Here's how the part is built. I have some questions about the finished solid (model axes, mm). A direction names the side the tool comes from. Give positions to 0.01 mm unless a question says otherwise; leave off trailing zeros. Loops run counter-clockwise (first coordinate to the right, second up) from the corner with the lowest first, then second, coordinate; pieces in that order, holes last. Notation, with made-up numbers: (-2.75, 36) - (45.25, 36) arc R13 cw to (45.25, 47) - close; hole circle Ø8 at (20.25, 25). An arc over 180 degrees is marked (long way). Return JSON: item names as keys, results as strings. Group by question number.
(1) For P1, Ø6, axis at x = 4.5, y = -23.5, coming from the +Z side; P2, Ø5, axis at x = -10.5, y = -39.5, coming from the +Z side; P3, Ø2.5, axis at y = -87.5, z = 10, coming from the -X side, each with a flat end and sliding along its axis, tell me the tip position at first contact or that it passes through.
(2) If we section it at D-D (y = 4.5): Please give me the cut outline in (x, z), then the cut area to 3 significant figures.
(3) If we section it at C-C (y = -60.5): Please give me the cut outline in (x, z).
(4) If we mould it in two halves opening along X, with no side actions, what happens to faces 1 (the cylindrical face through (-2.859, -21.203, 10.528)), 2 (the flat face through (-12.3, -10, -3.4)), 3 (the cylindrical face through (9.76, 34.65, -2.17)), 4 (the cylindrical face through (2.859, -21.203, 10.528))? For each: released by +X, released by -X, zero draft, split by the parting line, or undercut.
(5) I need wall thicknesses on probe 1 along Y at (x, z) = (8.75, 6); probe 2 along X at (y, z) = (-17, -0.75); probe 3 along Y at (x, z) = (-12, -8.75). Which ranges of each line are inside material? Lowest first, please. Write a range as [from, to].
(6) On a 3-axis mill with a long thin cutter (end or side, diameter ignored), from which of +Z, -Z, +X, -X, +Y, -Y can I reach the whole of each face in a straight line? I mean faces 5 (the cylindrical face through (-0.66, -0.14, -14.985)), 6 (the flat face through (4, -68, 10)), 7 (the cylindrical face through (7.606, -60.7, -9.92)), 8 (the flat face through (10, 10, -3)). Say none if no direction works.
(7) If we section it at A-A (z = 0): Please give me the cut outline in (x, y).
(8) If we section it at B-B (x = 5.75): Please give me the cut outline in (y, z).
```python
from build123d import *

# Parameters (mm, degrees)
F2_W     = 8
F2_H     = 4
F3_DEPTH = 90
F4_R     = 3.99999


# Not quite as in the source:
# - a fillet or chamfer is up to 0.001 mm smaller than in the source, because OpenCascade refuses the exact size


with BuildPart() as f1:
    # F0 (on Right) → F1 (revolve)
    with BuildSketch(Plane.YZ):
        Polygon((-110, 12.5), (-110, 0), (60, 0), (60, 10), (10, 10), (10, 15), (-10, 15), (-10, 12.5), align=None)
    revolve(axis=Axis((0, -25, 0), (0, -1, 0)))

    # F2 (on face) → F3 (cut)
    with BuildSketch(Plane.XZ.offset(110)):
        with Locations((0, 10.5)):
            Rectangle(F2_W, F2_H)
    extrude(amount=-F3_DEPTH, mode=Mode.SUBTRACT)

    # F4 (radius 4 in the source; OpenCascade refuses exactly that, so slightly less here)
    f4_edges = [f1.edges().sort_by_distance(p)[0] for p in [
        (-4, -20, 10.17136),
        (4, -20, 10.17136),
    ]]
    fillet(f4_edges, radius=F4_R)


solid = f1.part
```
Values:
{
 "1": {"P1": "z = 12.2", "P2": "z = 9.6", "P3": "x = -8.93"},
 "2": {"outline": "circle Ø30 at (0, 0)", "area": "707 mm2"},
 "3": {"outline": "(-4, 8.5) - (-4, 11.84) arc R12.5 ccw (long way) to (4, 11.84) - (4, 8.5) - close"},
 "4": {"face 1": "undercut", "face 2": "zero draft", "face 3": "split by the parting line", "face 4": "undercut"},
 "5": {"probe 1": "[-110, 10]", "probe 2": "[-12.48, 12.48]", "probe 3": "[-10, 10]"},
 "6": {"face 5": "+Y, -Y", "face 6": "+Z, -Y", "face 7": "-Y", "face 8": "+Y"},
 "7": {"outline": "(-15, -10) - (-12.5, -10) - (-12.5, -110) - (12.5, -110) - (12.5, -10) - (15, -10) - (15, 10) - (10, 10) - (10, 60) - (-10, 60) - (-10, 10) - (-15, 10) - close"},
 "8": {"outline": "(-110, -11.1) - (-10, -11.1) - (-10, -13.85) - (10, -13.85) - (10, -8.18) - (60, -8.18) - (60, 8.18) - (10, 8.18) - (10, 13.85) - (-10, 13.85) - (-10, 11.1) - (-110, 11.1) - close"}
}
